The model under review builds one solid part; all positions refer to its coordinate system, in mm. Face numbers are marked on the shaded views. Give positions to 0.01 mm unless a question says otherwise; leave off trailing zeros. Loops run counter-clockwise (first coordinate to the right, second up) from the corner with the lowest first, then second, coordinate; pieces in that order, holes last. Notation, with made-up numbers: M 43,-13.75 L 98,-13.75 A28 ccw 98,5.25 Z; hole C -11,65 d3. An arc over 180 degrees is marked long. Return JSON: item names as keys, results as strings. Group by question number.
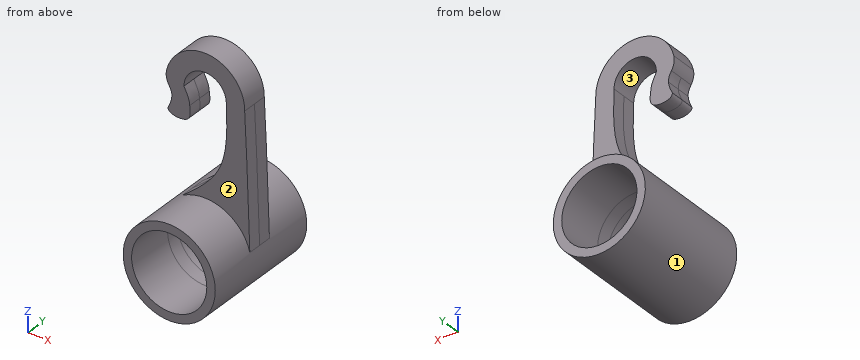
```python
from build123d import *

# Parameters (mm, degrees)
F0_R     = 13.5255
F1_DEPTH = 22.225
F2_DEPTH = 4.7625


with BuildPart() as f1:
    # F0 (on Front) → F1 (new body, symmetric)
    with BuildSketch(Plane.XZ):
        with BuildLine():
            ThreePointArc((16.0855769131, 3.991881464), (6.5567714231, 15.2213550893), (-8.1495274532, 14.4314276681))
            ThreePointArc((-8.1495274532, 14.4314276681), (-8.3550795629, -14.3134044779), (16.5735, 0))
            ThreePointArc((16.5735, 0), (16.4510670052, 2.0107950269), (16.0855769131, 3.991881464))
        make_face()
        Circle(F0_R, mode=Mode.SUBTRACT)
    extrude(amount=F1_DEPTH, both=True)

    # F0 (on Front) → F2 (join, symmetric)
    with BuildSketch(Plane.XZ):
        with BuildLine():
            ThreePointArc((16.0855769131, 3.991881464), (6.5567714231, 15.2213550893), (-8.1495274532, 14.4314276681))
            ThreePointArc((-8.1495274532, 14.4314276681), (-8.3550795629, -14.3134044779), (16.5735, 0))
            ThreePointArc((16.5735, 0), (16.4510670052, 2.0107950269), (16.0855769131, 3.991881464))
        make_face()
        Circle(F0_R, mode=Mode.SUBTRACT)
        with BuildLine():
            add(Edge.make_bspline(
                [(7.6196315943, 52.0585709196), (7.9073561804, 43.8512833929), (8.4668828165, 27.9749976478), (-2.735262235, 18.8402392219), (-8.1495274532, 14.4314276681)],
                knots=[0, 0, 0, 0, 0.5168803488, 1, 1, 1, 1], degree=3))
            ThreePointArc((-8.1495274532, 14.4314276681), (6.5567714231, 15.2213550893), (16.0855769131, 3.991881464))
            add(Edge.make_bspline(
                [(14.2219077444, 51.8895407599), (14.4256822763, 47.7682077132), (14.9759634895, 37.2014626867), (15.653478831, 16.5725180559), (16.0855769131, 3.991881464)],
                knots=[0, 0, 0, 0, 0.3900119934, 1, 1, 1, 1], degree=3))
            ThreePointArc((14.2219077444, 51.8895407599), (1.6964946006, 66.2559672798), (-13.8750644733, 55.2647556367))
            ThreePointArc((-13.8750644733, 55.2647556367), (-13.937377269, 52.7814096229), (-13.0421995878, 50.4641812725))
            add(Edge.make_bspline(
                [(-13.0421995878, 50.4641812725), (-12.3253096001, 49.3346329312), (-11.8330637514, 48.1700341933), (-12.0167843997, 46.8999668956)],
                knots=[0.0832842621, 0.0832842621, 0.0832842621, 0.0832842621, 0.2506068983, 0.2506068983, 0.2506068983, 0.2506068983], degree=3))
            add(Edge.make_bspline(
                [(-12.0167843975, 46.8999668404), (-11.9685081536, 45.6929371066), (-12.6474764459, 44.2057904092), (-13.352232419, 42.7222704399)],
                knots=[0.6168006178, 0.6168006178, 0.6168006178, 0.6168006178, 1, 1, 1, 1], degree=3))
            add(Edge.make_bspline(
                [(-13.352232419, 42.7222704399), (-13.3723404879, 42.3903517549), (-13.0294229695, 40.5231715226), (-8.3379146473, 40.1111053623), (-6.5978615691, 41.1531167984)],
                knots=[0.4383260576, 0.4383260576, 0.4383260576, 0.4383260576, 0.4904587097, 0.7585657185, 0.7585657185, 0.7585657185, 0.7585657185], degree=3))
            add(Edge.make_bspline(
                [(-5.5660903454, 46.2477467954), (-5.5050556705, 44.6482001002), (-5.9652585792, 42.9216600644), (-6.5978615691, 41.1531167984)],
                knots=[0.4687776215, 0.4687776215, 0.4687776215, 0.4687776215, 0.8242974336, 0.8242974336, 0.8242974336, 0.8242974336], degree=3))
            add(Edge.make_bspline(
                [(-7.62, 52.1335), (-6.6332844065, 50.2451802325), (-5.6465688131, 48.356860465), (-5.5660903454, 46.2477467954)],
                knots=[0, 0, 0, 0, 0.4687776215, 0.4687776215, 0.4687776215, 0.4687776215], degree=3))
            ThreePointArc((-7.62, 52.1335), (0.037464993, 59.753407898), (7.6196315943, 52.0585709196))
        make_face()
        with BuildLine():
            add(Edge.make_bspline(
                [(-6.5978615691, 41.1531167984), (-6.5808454576, 41.1633067076), (-5.0331676538, 42.1138674091), (-5.3010837075, 44.1920912662), (-5.5660903454, 46.2477467954)],
                knots=[0.7585657185, 0.7585657185, 0.7585657185, 0.7585657185, 0.7611875574, 1, 1, 1, 1], degree=3))
            add(Edge.make_bspline(
                [(-5.5660903454, 46.2477467954), (-5.5050556705, 44.6482001002), (-5.9652585792, 42.9216600644), (-6.5978615691, 41.1531167984)],
                knots=[0.4687776215, 0.4687776215, 0.4687776215, 0.4687776215, 0.8242974336, 0.8242974336, 0.8242974336, 0.8242974336], degree=3))
        make_face()
    extrude(amount=F2_DEPTH, both=True)


solid = f1.part
```
(1) Add section D-D (x = 2). Count the separate pieces of the cut face and the enclosed holes in it, and give its area (3 significant figures).
(2) Add section C-C (y = -18). Write out the cut boundary in (x, z), and give its area (3 significant figures).
(3) For probe 1 along Z at (x, y) = (0, -14); probe 2 along Z at (x, y) = (0, 1); probe 3 along Z at (x, y) = (-4, -16), list the stretches that pass through material, from the lowest coordinate up.
(4) Add section A-A (z = 0). Write out the cut boundary in (x, y) (1 decimal), and give its area (3 significant figures).
(5) Mouldability with a two-part tool opening along X and no side actions: class the marked faces 1, 2 and 3 as released by +X, released by -X, zero draft, split by the parting line, or undercut.
(6) Add section B-B (x = 10.5). Write out the cut boundary in (y, z) (1 decimal).
(7) For pin 1 (12 mm diameter, centred on y = -8.5, z = 38.5, fed in from +X); pin 2 (4 mm diameter, centred on y = -10.5, z = 15, fed in from +X); pin 3 (10 mm diameter, centred on y = 3, z = 26.5, fed in from -X); pin 4 (16 mm diameter, centred on x = 0, z = 0, fed in from +Y), all flat-tipped, find the tip position at first contact; note any pin that passes through.
Verdict:
{
 "1": {"separate pieces": "3", "enclosed holes": "0", "area": "408 mm²"},
 "2": {"outline": "C 0,0 d33.15; hole C 0,0 d27.05", "area": "288 mm²"},
 "3": {"probe 1": "z = -16.57 to -13.53, 13.53 to 16.57", "probe 2": "z = -16.57 to -13.53, 13.53 to 21.63, 59.75 to 66.36", "probe 3": "z = -16.08 to -12.92, 12.92 to 16.08"},
 "4": {"outline": "M -16.6,-22.2 L -13.5,-22.2 L -13.5,22.2 L -16.6,22.2 Z; M 13.5,-22.2 L 16.6,-22.2 L 16.6,22.2 L 13.5,22.2 Z", "area": "271 mm²"},
 "5": {"face 1": "split by the parting line", "face 2": "zero draft", "face 3": "undercut"},
 "6": {"outline": "M -22.2,-12.8 L 22.2,-12.8 L 22.2,-8.5 L -22.2,-8.5 Z; M -22.2,8.5 L 22.2,8.5 L 22.2,12.8 L 4.8,12.8 L 4.8,61.7 L -4.8,61.7 L -4.8,12.8 L -22.2,12.8 Z"},
 "7": {"pin 1": "stops at x = 15.04", "pin 2": "stops at x = 10.28", "pin 3": "stops at x = -0.12", "pin 4": "passes through"}
}
